Here's how the part is built. I have some questions about the finished solid (model axes, mm). Face numbers are marked on the shaded views. Coordinates: 2 decimals unless noted, no trailing zeros. Order: outer loops, then holes, each group sorted by start corner. A loop starts at its lowest first (then second) coordinate and runs counter-clockwise, first axis right, second up. Notation, with made-up numbers: (-35, 83) - (-23, 83) arc R26 ccw to (-23, 99) - close; hole circle Ø5 at (-18, 10.25). An arc over 180 degrees is marked (long way). Answer in a Markdown table with one row per item. Add a question column.
Item 1: I want a section at B-B (y = 0). Please give me the cut outline in (x, z).
Item 2: I want a section at A-A (x = 33). Please give me the cut outline in (y, z), plus the area to 3 significant figures.
Item 3: If I drill on line 1 along Y through (x, z) = (33, 7); line 2 along X through (y, z) = (0.1, 7.5); line 3 along X through (y, z) = (-1.05, 6.25), over which ranges is the centre line in solid material (lowest first)? Write a range as from..to.
Item 4: I want a section at C-C (z = 7.25). Please give me the cut outline in (x, y).
Item 5: Thinking about a two-plate mould opening in X: for the marked faces 1 and 2, which applies, +X half, -X half, draft (parallel to the pull), parting line (faces both ways), or undercut?
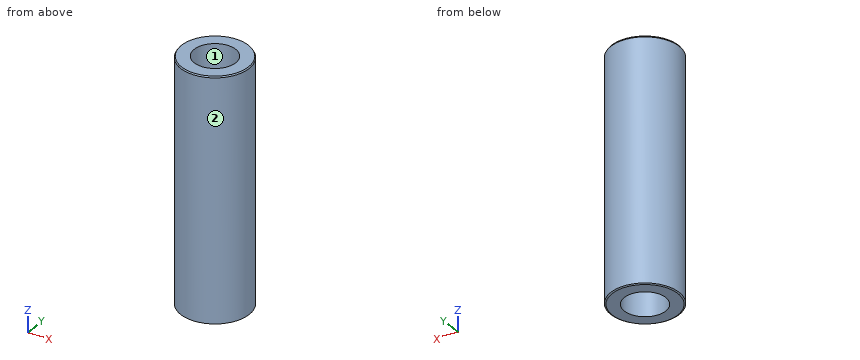
```python
from build123d import *
from OCP.BRepFilletAPI import BRepFilletAPI_MakeChamfer

# Parameters (mm, degrees)
SKETCH1_R           = 2.55
BOSS_EXTRUDE1_DEPTH = 18
CUT_EXTRUDE1_REACH  = 41.929
SKETCH3_R           = 1.55
CHAMFER1_SIZE       = 0.1
CHAMFER1_SIZE2      = 0.057735027


with BuildPart() as part:
    # Sketch1 → Boss-Extrude1 (new body)
    with BuildSketch(Plane.XY):
        with Locations((33, 0)):
            Circle(SKETCH1_R)
    extrude(amount=BOSS_EXTRUDE1_DEPTH)

    # Sketch3 → Cut-Extrude1 (cut, up to next)
    with BuildSketch(Plane.XY.offset(18), mode=Mode.PRIVATE) as cut_extrude1_sk1:
        with Locations((33, 0)):
            Circle(SKETCH3_R)
    cut_extrude1_tool1 = extrude(cut_extrude1_sk1.sketch, amount=-CUT_EXTRUDE1_REACH, mode=Mode.PRIVATE) & part.part
    add(cut_extrude1_tool1.solids().sort_by_distance((33, 0, 18))[0], mode=Mode.SUBTRACT)

    # Chamfer1: one chamfer whose edges measure the first distance from different faces: ONE call of the kernel's chamfer builder (chamfer() names one face for all edges)
    chamfer1_edges_1 = [part.edges().sort_by_distance(p)[0] for p in [
        (30.45, 0, 0),
    ]]
    chamfer1_side_1 = [part.faces().sort_by_distance(p)[0] for p in [
        (30.522124892, 0, 0),
    ]]
    chamfer1_edges_2 = [part.edges().sort_by_distance(p)[0] for p in [
        (30.45, 0, 18),
    ]]
    chamfer1_side_2 = [part.faces().sort_by_distance(p)[0] for p in [
        (30.45, 0, 9),
    ]]
    chamfer1 = BRepFilletAPI_MakeChamfer(part.part.solid().wrapped)
    for e in chamfer1_edges_1:
        chamfer1.Add(CHAMFER1_SIZE, CHAMFER1_SIZE2, e.wrapped, chamfer1_side_1[0].wrapped)  # the first distance lies on this face
    for e in chamfer1_edges_2:
        chamfer1.Add(CHAMFER1_SIZE, CHAMFER1_SIZE2, e.wrapped, chamfer1_side_2[0].wrapped)  # the first distance lies on this face
    add(Compound.cast(chamfer1.Shape()), mode=Mode.REPLACE)


solid = part.part
```
Values follow:
| question | item | result |
|---|---|---|
| 1 | outline | (30.45, 0.06) - (30.55, 0) - (31.45, 0) - (31.45, 18) - (30.51, 18) - (30.45, 17.9) - close; (34.55, 0) - (35.45, 0) - (35.55, 0.06) - (35.55, 17.9) - (35.49, 18) - (34.55, 18) - close |
| 2 | outline | (-2.55, 0.06) - (-2.45, 0) - (-1.55, 0) - (-1.55, 18) - (-2.49, 18) - (-2.55, 17.9) - close; (1.55, 0) - (2.45, 0) - (2.55, 0.06) - (2.55, 17.9) - (2.49, 18) - (1.55, 18) - close |
| 2 | area | 36.0 mm^2 |
| 3 | line 1 | y = -2.55..-1.55, 1.55..2.55 |
| 3 | line 2 | x = 30.45..31.45, 34.55..35.55 |
| 3 | line 3 | x = 30.68..31.86, 34.14..35.32 |
| 4 | outline | circle Ø5.1 at (33, 0); hole circle Ø3.1 at (33, 0) |
| 5 | face 1 | undercut |
| 5 | face 2 | parting line |
